The listing builds one solid part. Answer for the finished solid, in the listing's coordinates (mm). A direction names the side the tool comes from. Round coordinates to 2 decimals unless told otherwise and drop trailing zeros. Write each loop counter-clockwise with the first axis right and the second up, starting at its lowest first coordinate (ties: lowest second). Pieces come first, ordered by that corner, then holes. Notation, with made-up numbers: (4, -20) - (29, -20) arc R16 cw to (29, -2) - close; hole circle Ø10 at (33, 77.25). An arc over 180 degrees is marked (long way). Answer in a Markdown table with one row per item.
from build123d import *

# Parameters (mm, degrees)
SKETCH1_R          = 15.875
RAWSTOCK_DEPTH     = 194.6402
SKETCH10_R         = 12.7
FACINGOP_DEPTH     = 23.1902
RELIEFHOLE_D       = 12.7
RELIEFHOLE_DEPTH   = 92.075
RELIEFHOLE_TIP     = 3.815464931
WIRESHOLE_D        = 15.875
WIRESHOLE_DEPTH    = 115.2652
WIRESHOLE_TIP      = 4.769331164
SKETCH6_OUTSIDE_W  = 73.7
SKETCH6_OUTSIDE_H  = 73.7
SKETCH6_OUTSIDE_R  = 12.7
SHAFTDIAM_DEPTH    = 124.7902
SKETCH7_OUTSIDE_W  = 69.196
SKETCH7_OUTSIDE_H  = 69.196
SKETCH7_OUTSIDE_R  = 11.938
GROOVE_DEPTH       = 1.190625
SKETCH8_OUTSIDE_W  = 69.196
SKETCH8_OUTSIDE_H  = 69.196
SKETCH8_OUTSIDE_R  = 6.35
ENCODERSHAFT_DEPTH = 66.675
SKETCH12_R         = 3.96875
SKETCH12_R_2       = 4.7625
HOLES_TOP_DEPTH    = 29.575
SLIPRINGHOLE_D     = 4.7625
SLIPRINGHOLE_DEPTH = 25.4
SLIPRINGHOLE_TIP   = 1.430799349


with BuildPart() as part:
    # Sketch1 → RawStock (new body)
    with BuildSketch(Plane.XY):
        Circle(SKETCH1_R)
    extrude(amount=RAWSTOCK_DEPTH)

    # Sketch10 → FacingOp (cut)
    with BuildSketch(Plane.XY.offset(194.6402)):
        Circle(SKETCH10_R)
    extrude(amount=-FACINGOP_DEPTH, mode=Mode.SUBTRACT)

    # ReliefHole
    with Locations(Plane.XY.offset(194.6402)):
        with Locations((0, 0)):
            Hole(RELIEFHOLE_D / 2, depth=RELIEFHOLE_DEPTH)
            with Locations((0, 0, -(RELIEFHOLE_DEPTH + RELIEFHOLE_TIP / 2))):  # 118° drill point
                Cone(0, RELIEFHOLE_D / 2, RELIEFHOLE_TIP, mode=Mode.SUBTRACT)

    # WiresHole
    with Locations(Plane.XY.offset(194.6402)):
        with Locations((0, 0)):
            Hole(WIRESHOLE_D / 2, depth=WIRESHOLE_DEPTH)
            with Locations((0, 0, -(WIRESHOLE_DEPTH + WIRESHOLE_TIP / 2))):  # 118° drill point
                Cone(0, WIRESHOLE_D / 2, WIRESHOLE_TIP, mode=Mode.SUBTRACT)

    # Sketch6 outside → ShaftDiam (cut)
    with BuildSketch(Plane.XY.offset(194.6402)):
        Rectangle(SKETCH6_OUTSIDE_W, SKETCH6_OUTSIDE_H)
        Circle(SKETCH6_OUTSIDE_R, mode=Mode.SUBTRACT)
    extrude(amount=-SHAFTDIAM_DEPTH, mode=Mode.SUBTRACT)

    # Sketch7 outside → Groove (cut)
    with BuildSketch(Plane.XY.offset(130.175)):
        Rectangle(SKETCH7_OUTSIDE_W, SKETCH7_OUTSIDE_H)
        Circle(SKETCH7_OUTSIDE_R, mode=Mode.SUBTRACT)
    extrude(amount=GROOVE_DEPTH, mode=Mode.SUBTRACT)

    # Sketch8 outside → EncoderShaft (cut)
    with BuildSketch(Plane(origin=(0, 0, 0), x_dir=(-1, 0, 0), z_dir=(0, 0, -1))):
        Rectangle(SKETCH8_OUTSIDE_W, SKETCH8_OUTSIDE_H)
        Circle(SKETCH8_OUTSIDE_R, mode=Mode.SUBTRACT)
    extrude(amount=-ENCODERSHAFT_DEPTH, mode=Mode.SUBTRACT)

    # Sketch12 → Holes_Top (cut, through all)
    with BuildSketch(Plane(origin=(-12.7, 0, 0), x_dir=(0, 1, 0), z_dir=(-1, 0, 0))):
        with Locations((0, -161.925)):
            Circle(SKETCH12_R)
        with Locations((0, -147.6375)):
            Circle(SKETCH12_R_2)
    extrude(amount=-HOLES_TOP_DEPTH, mode=Mode.SUBTRACT)

    # SlipRingHole
    with Locations(Plane(origin=(0, 0, 66.675), x_dir=(-1, 0, 0), z_dir=(0, 0, -1))):
        with Locations((0, -8.73125)):
            Hole(SLIPRINGHOLE_D / 2, depth=SLIPRINGHOLE_DEPTH)
            with Locations((0, 0, -(SLIPRINGHOLE_DEPTH + SLIPRINGHOLE_TIP / 2))):  # 118° drill point
                Cone(0, SLIPRINGHOLE_D / 2, SLIPRINGHOLE_TIP, mode=Mode.SUBTRACT)


solid = part.part
(1) Find the intervals of material crossed by line 1 (Z direction, x = -9, y = 0) (3 decimals); line 2 (Z direction, x = 9, y = 1) (3 decimals); line 3 (Y direction, x = 0, z = 153), in increasing order.
Checked values:
| item | result |
|---|---|
| line 1 | z = 66.675 to 142.875, 152.4 to 157.956, 165.894 to 171.45 |
| line 2 | z = 66.675 to 142.981, 152.294 to 158.084, 165.766 to 171.45 |
| line 3 | y = -12.7 to -7.94, 7.94 to 12.7 |
(2) For a pull along Z with two mould halves and no side action, classify faces 1 (the flat face through (0, 0, 0)), 2 (the cylindrical face through (-9.57, 4.543, 146.207)), 3 (the flat face through (-7, 11, 69.85)) as pulls with the +Z half, pulls with the -Z half, needs draft (parallel to the pull), parting line crosses it, or undercut.
Checked values:
| item | result |
|---|---|
| face 1 | pulls with the -Z half |
| face 2 | undercut |
| face 3 | pulls with the +Z half |
(3) Section B-B (z = 115.5) is taken. Give the vertices of the cut face in (x, y) (1 decimal).
Checked values:
| item | result |
|---|---|
| outline | circle Ø25.4 at (0, 0); hole circle Ø15.9 at (0, 0) |
(4) Section C-C (z = 55.5) is taken. Give the vertices of the cut face in (x, y).
Checked values:
| item | result |
|---|---|
| outline | circle Ø12.7 at (0, 0) |
(5) Flat-ended cylindrical pins translate along their axes: pin 1 (15 mm diameter, centred on y = 0, z = 147.64, fed in from -X); pin 2 (8 mm diameter, centred on y = 2, z = 153.5, fed in from +X); pin 3 (1.5 mm diameter, centred on y = -12, z = 99.5, fed in from -X). Find the tip coordinate at first contact, or state that the pin passes through.
Checked values:
| item | result |
|---|---|
| pin 1 | stops at x = -12.7 |
| pin 2 | stops at x = 12.7 |
| pin 3 | stops at x = -5.89 |
(6) Section A-A (x = -9.5) is taken. State how many separate pieces and enclosed holes the cut face has, and give its area (3 significant figures).
Checked values:
| item | result |
|---|---|
| separate pieces | 1 |
| enclosed holes | 2 |
| area | 1,670 mm2 |
(7) For faces 4 (the flat face through (-7, 0, 66.675)), 5 (the flat face through (-0.2, -8.3, 171.45)), 6 (the cylindrical face through (9.746, 3.785, 160.733)), 7 (the cylindrical face through (-2.75, -12.4, 100.43)), 8 (the flat face through (11.2, -4.6, 131.366)), determine the directions among +Z, -Z, +X, -X, +Y, -Y from which every point of the face is accessible in a straight line to the end or side of a thin tool.
Checked values:
| item | result |
|---|---|
| face 4 | -Z |
| face 5 | +Z, +X, -X, +Y, -Y |
| face 6 | +X, -X |
| face 7 | +Z |
| face 8 | none |
